Verification items for the finished model (mm, model axes). Face numbers are marked on the shaded views. Give positions to 0.01 mm unless a question says otherwise; leave off trailing zeros. Write each loop counter-clockwise with the first axis right and the second up, starting at its lowest first coordinate (ties: lowest second). Pieces come first, ordered by that corner, then holes. Notation, with made-up numbers: (86, 70) - (125, 70) arc R21 cw to (125, 79) - close; hole circle Ø7 at (25, 5). An arc over 180 degrees is marked (long way). Answer as a JSON object with one key per item and string values. Group by question number.
Item 1: Go/stop test with flat-tipped pins: pin 1 (1 mm diameter, centred on y = 1, z = 2, fed in from -X); pin 2 (4 mm diameter, centred on x = 0, y = 0, fed in from +Z); pin 3 (1 mm diameter, centred on x = 3, z = 2.5, fed in from -Y). Record where each tip stops, or that it passes through.
Item 2: Scan lines: line 1 along Y through (x, z) = (0, 0.45); line 2 along X through (y, z) = (-1.5, 1.15); line 3 along Y through (x, z) = (-0.75, 2.25). Record each from-to range of solid material in increasing order. Write a range as [from, to].
Item 3: Sectioned sample at C-C, the plane z = 1.2. Record the boundary of the cut face in (x, y).
Item 4: Sectioned sample at A-A, the plane y = 0. Record the boundary of the cut face in (x, z).
Item 5: Sectioned sample at D-D, the plane z = 2.35. Record the boundary of the cut face in (x, y), and give its area (3 significant figures).
Item 6: Draft check along Y on the marked faces 1, 2 and 3. Enter one of: +Y half, -Y half, draft (parallel to the pull), parting line (faces both ways), or undercut.
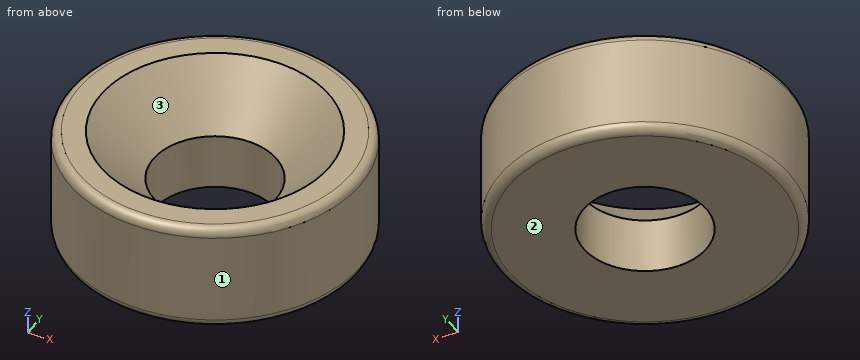
Autodesk Fusion 360 part; units mm, degrees
sketch "Sketch1" plane through (0, 0, 0) normal (0, 0, 1) x (1, 0, 0)
  circle A0 centre (0, 0) radius 4
  dimension "d1" = 8
extrude "Extrude1" add sketch "Sketch1" along normal blind 3
hole "Hole1" at (0, 0, 3) direction (0, 0, -1) diameter 3.4 depth 8 tip angle 118 countersink diameter 6.3 countersink angle 90
fillet "Fillet1" radius 0.25 2 edges at (-3.7293, -1.4465, 0) (-3.7293, -1.4465, 3)
Geometry check:
{
 "1": {"pin 1": "x = -3.97", "pin 2": "z = 1.85", "pin 3": "y = -3.12"},
 "2": {"line 1": "[-4, -1.7], [1.7, 4]", "line 2": "[-3.71, -0.8], [0.8, 3.71]", "line 3": "[-3.93, -2.28], [2.28, 3.93]"},
 "3": {"outline": "circle Ø8 at (0, 0); hole circle Ø3.4 at (0, 0)"},
 "4": {"outline": "(-4, 0.25) arc R0.25 ccw to (-3.75, 0) - (-1.7, 0) - (-1.7, 1.55) - (-3.15, 3) - (-3.75, 3) arc R0.25 ccw to (-4, 2.75) - close; (1.7, 0) - (3.75, 0) arc R0.25 ccw to (4, 0.25) - (4, 2.75) arc R0.25 ccw to (3.75, 3) - (3.15, 3) - (1.7, 1.55) - close"},
 "5": {"outline": "circle Ø8 at (0, 0); hole circle Ø5 at (0, 0)", "area": "30.6 mm^2"},
 "6": {"face 1": "parting line", "face 2": "draft", "face 3": "undercut"}
}
